```python
from build123d import *

# Parameters (mm, degrees)
EXTRUDE_1_DEPTH     = 100
SKETCH_3_R          = 10
EXTRUDE_2_DEPTH     = 20
SKETCH_4_W          = 40
SKETCH_4_H          = 40
CUT_EXTRUDE_1_DEPTH = 12


with BuildPart() as part:
    # Эскиз1 → Бобышка-Вытянуть1 (new body)
    with BuildSketch(Plane.XY):
        Polygon((0, 0), (0, 20), (70, 20), (70, 0), (60, 0), (60, 8), (10, 8), (10, 0), align=None)
    extrude(amount=EXTRUDE_1_DEPTH)

    # Эскиз3 → Бобышка-Вытянуть2 (add)
    with BuildSketch(Plane(origin=(0, 0, 0), x_dir=(-1, 0, 0), z_dir=(0, 0, -1))):
        with BuildLine():
            Line((-60, 20), (-60, 35))
            ThreePointArc((-60, 35), (-35, 60), (-10, 35))
            Line((-10, 35), (-10, 20))
            Line((-10, 20), (-60, 20))
        make_face()
        with Locations((-35, 35)):
            Circle(SKETCH_3_R, mode=Mode.SUBTRACT)
    extrude(amount=-EXTRUDE_2_DEPTH)

    # Эскиз4 → Вырез-Вытянуть1 (cut)
    with BuildSketch(Plane(origin=(0, 20, 0), x_dir=(1, 0, 0), z_dir=(0, 1, 0))):
        with Locations((35, -70)):
            Rectangle(SKETCH_4_W, SKETCH_4_H)
    extrude(amount=-CUT_EXTRUDE_1_DEPTH, mode=Mode.SUBTRACT)


solid = part.part
```
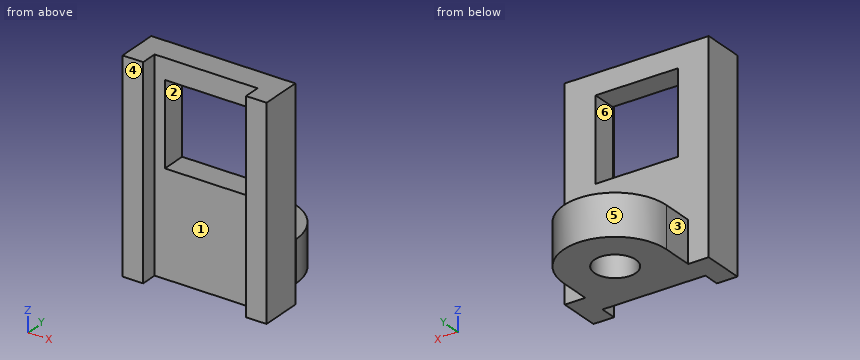
Geometry: final body of the model. Coordinates: model frame, mm. Face numbers are marked on the shaded views. A direction names the side the tool comes from. Round coordinates to 2 decimals unless told otherwise and drop trailing zeros. Loops run counter-clockwise (first coordinate to the right, second up) from the corner with the lowest first, then second, coordinate; pieces in that order, holes last. Notation, with made-up numbers: (34.25, 24.25) -> (83.25, 24.25) arc R20 ccw to (83.25, 55.25) -> close; hole circle Ø3 at (-21.5, 78.5). An arc over 180 degrees is marked (long way). Use one line per item in the form item = value. Start each with the question number.
1) Access query for the marked faces 5 and 6. Directions: +Z, -Z, +X, -X, +Y, -Y. A direction counts if a zero-diameter tool reaches every point of the face in a straight line with its end or side. Return the directions, or none.
2) Line query: L1, parallel to X at y = 15.5, z = 87; L2, parallel to Z at x = 37, y = 19.5; L3, parallel to Y at x = 35, z = 10. Output: solid intervals per line, ascending.
3) Section A-A on x = 35. Output: boundary loops of the cut face in (y, z), then the cut area to 3 significant figures.
4) Section D-D on x = 52. Output: boundary loops of the cut face in (y, z), then the cut area to 3 significant figures.
5) First-contact query: P1, Ø12, axis at x = 24.5, y = 39.5, coming from the +Z side; P2, Ø6, axis at x = 54.5, z = 35, coming from the +Y side. Flat tips, straight axial feed; report the tip coordinate or a pass-through.
6) Section B-B on z = 12.5. Output: boundary loops of the cut face in (x, y), then the cut area to 3 significant figures.
7) Section C-C on z = 77. Output: boundary loops of the cut face in (x, y).
8) Draft query along X for the marked faces 1, 2, 3 and 4. Return one class per face: released by +X, released by -X, zero draft, split by the parting line, or undercut.
Response:
q1.face_5 = +Z, -Z, +Y
q1.face_6 = +Y, -Y
q2.L1 = 0 to 15, 55 to 70
q2.L2 = 0 to 50, 90 to 100
q2.L3 = 8 to 25, 45 to 60
q3.outline = (8, 0) -> (25, 0) -> (25, 20) -> (20, 20) -> (20, 50) -> (8, 50) -> close; (8, 90) -> (20, 90) -> (20, 100) -> (8, 100) -> close; (45, 0) -> (60, 0) -> (60, 20) -> (45, 20) -> close
q3.area = 1,120 mm^2
q4.outline = (8, 0) -> (53.33, 0) -> (53.33, 20) -> (20, 20) -> (20, 50) -> (8, 50) -> close; (8, 90) -> (20, 90) -> (20, 100) -> (8, 100) -> close
q4.area = 1,390 mm^2
q5.P1 = 20
q5.P2 = 20
q6.outline = (0, 0) -> (10, 0) -> (10, 8) -> (60, 8) -> (60, 0) -> (70, 0) -> (70, 20) -> (60, 20) -> (60, 35) arc R25 ccw to (10, 35) -> (10, 20) -> (0, 20) -> close; hole circle Ø20 at (35, 35)
q6.area = 2,420 mm^2
q7.outline = (0, 0) -> (10, 0) -> (10, 8) -> (15, 8) -> (15, 20) -> (0, 20) -> close; (55, 8) -> (60, 8) -> (60, 0) -> (70, 0) -> (70, 20) -> (55, 20) -> close
q8.face_1 = undercut
q8.face_2 = undercut
q8.face_3 = released by -X
q8.face_4 = zero draft
